```python
from build123d import *

# Parameters (mm, degrees)
SKETCH_13_W         = 280
SKETCH_13_H         = 14.842907488
EXTRUDE_14_DEPTH    = 20
SKETCH_13_W_2       = 18.151554109
SKETCH_13_H_2       = 185
EXTRUDE_14_2_DEPTH  = 20
SKETCH_13_H_3       = 15.157092512
EXTRUDE_14_3_DEPTH  = 20
SKETCH_13_W_3       = 16.848445891
EXTRUDE_14_4_DEPTH  = 20
SKETCH_29_W         = 18.151554109
SKETCH_29_H         = 14.842907488
SKETCH_29_W_2       = 16.848445891
SKETCH_29_H_2       = 15.157092512
EXTRUDE_15_DEPTH    = 400
EXTRUDE_START       = -16.848446
SKETCH_33_W         = 13.5
SKETCH_33_H         = 185
EXTRUDE_16_DEPTH    = 16.848446
EXTRUDE_START_2     = -18.151554
SKETCH_32_W         = 13.5
SKETCH_32_H         = 185
EXTRUDE_17_DEPTH    = 18.151554
EXTRUDE_START_3     = -14.842907
SKETCH_31_W         = 280
SKETCH_31_H         = 13.5
EXTRUDE_18_DEPTH    = 14.842907
SKETCH_30_W         = 280
SKETCH_30_H         = 13.5
EXTRUDE_19_DEPTH    = 15.15709
SKETCH_34_R         = 7
CUT_EXTRUDE_1_DEPTH = 20


with BuildPart() as part:
    # Sketch 13 → Extrude 14 (new body)
    with BuildSketch(Plane.XY):
        with Locations((158.151554109, 207.578546256)):
            Rectangle(SKETCH_13_W, SKETCH_13_H)
    extrude(amount=EXTRUDE_14_DEPTH)



with BuildPart() as body_2:
    # Sketch 13 → Extrude 14 2 (new body)
    with BuildSketch(Plane.XY):
        with Locations((9.075777055, 107.657092512)):
            Rectangle(SKETCH_13_W_2, SKETCH_13_H_2)
    extrude(amount=EXTRUDE_14_2_DEPTH)


with BuildPart() as body_3:
    # Sketch 13 → Extrude 14 3 (new body)
    with BuildSketch(Plane.XY):
        with Locations((158.151554109, 7.578546256)):
            Rectangle(SKETCH_13_W, SKETCH_13_H_3)
    extrude(amount=EXTRUDE_14_3_DEPTH)


with BuildPart() as body_4:
    # Sketch 13 → Extrude 14 4 (new body)
    with BuildSketch(Plane.XY):
        with Locations((306.575777055, 107.657092512)):
            Rectangle(SKETCH_13_W_3, SKETCH_13_H_2)
    extrude(amount=EXTRUDE_14_4_DEPTH)


with BuildPart() as part_1:
    add(part.part)

    add(body_2.part)  # Extrude 15 merges body 2

    add(body_3.part)  # Extrude 15 merges body 3

    add(body_4.part)  # Extrude 15 merges body 4
    # Sketch 29 → Extrude 15 (add)
    with BuildSketch(Plane.XY):
        with Locations((9.075777055, 207.578546256)):
            Rectangle(SKETCH_29_W, SKETCH_29_H)
        with Locations((306.575777055, 207.578546256)):
            Rectangle(SKETCH_29_W_2, SKETCH_29_H)
        with Locations((9.075777055, 7.578546256)):
            Rectangle(SKETCH_29_W, SKETCH_29_H_2)
        with Locations((306.575777055, 7.578546256)):
            Rectangle(SKETCH_29_W_2, SKETCH_29_H_2)
    extrude(amount=EXTRUDE_15_DEPTH)

    # Sketch 33 → Extrude 16 (add)
    with BuildSketch(Plane(origin=(315, 0, 0), x_dir=(0, 0, -1), z_dir=(1, 0, 0)).offset(EXTRUDE_START)):
        with Locations((-323.114974864, 107.657092512)):
            Rectangle(SKETCH_33_W, SKETCH_33_H)
    extrude(amount=EXTRUDE_16_DEPTH)

    # Sketch 32 → Extrude 17 (add)
    with BuildSketch(Plane.ZY.offset(EXTRUDE_START_2)):
        with Locations((323.114974864, 107.657092512)):
            Rectangle(SKETCH_32_W, SKETCH_32_H)
    extrude(amount=EXTRUDE_17_DEPTH)

    # Sketch 31 → Extrude 18 (add)
    with BuildSketch(Plane(origin=(0, 215, 0), x_dir=(1, 0, 0), z_dir=(0, 1, 0)).offset(EXTRUDE_START_3)):
        with Locations((158.151554109, -345.610164736)):
            Rectangle(SKETCH_31_W, SKETCH_31_H)
    extrude(amount=EXTRUDE_18_DEPTH)

    # Sketch 30 → Extrude 19 (add)
    with BuildSketch(Plane.XZ):
        with Locations((158.151554109, 345.610164736)):
            Rectangle(SKETCH_30_W, SKETCH_30_H)
    extrude(amount=-EXTRUDE_19_DEPTH)

    # Sketch 34 → Cut-Extrude 1 (cut)
    with BuildSketch(Plane(origin=(0, 0, 0), x_dir=(-1, 0, 0), z_dir=(0, 0, -1))):
        with Locations((-279.91, 207.578546256)):
            Circle(SKETCH_34_R)
        with Locations((-279.91, 7.566753944)):
            Circle(SKETCH_34_R)
        with Locations((-28.27, 207.578546256)):
            Circle(SKETCH_34_R)
        with Locations((-28.27, 7.566753944)):
            Circle(SKETCH_34_R)
    extrude(amount=-CUT_EXTRUDE_1_DEPTH, mode=Mode.SUBTRACT)


solid = part_1.part
```
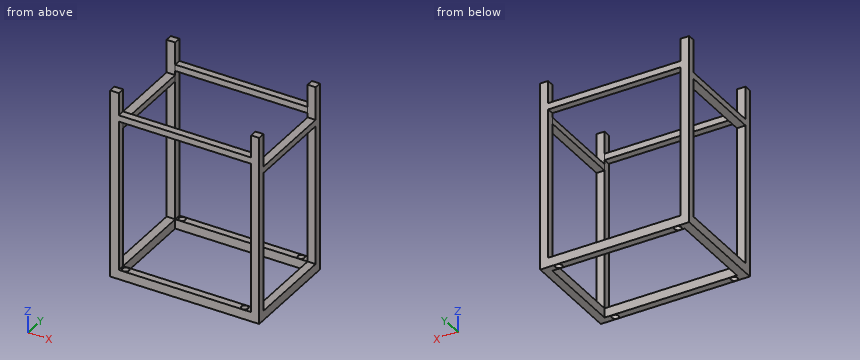
Source: CAD feature listing. Evaluate the final solid. Frame: model axes, mm. Round coordinates to 2 decimals unless told otherwise and drop trailing zeros. Loops run counter-clockwise (first coordinate to the right, second up) from the corner with the lowest first, then second, coordinate; pieces in that order, holes last. Notation, with made-up numbers: M 36.5,3 L 77.5,3 A20 cw 77.5,27 Z; hole C 26.5,-15.5 d3. An arc over 180 degrees is marked long. Use a Markdown table: item, result. Add a question column.
1. Cut plane A-A, the plane x = 28.27. Output: boundary loops of the cut face in (y, z), and give its area (3 significant figures).
2. Cut plane C-C, the plane y = 97.5. Output: boundary loops of the cut face in (x, z), and give its area (3 significant figures).
3. Ray query, line 1 along Y through (x, z) = (28.27, 6.5); line 2 along Y through (x, z) = (284.5, 352); line 3 along Z through (x, y) = (191.5, 14.5). Return the intervals inside material, ascending. Write a range as [from, to].
4. Cut plane B-B, the plane z = 245. Output: boundary loops of the cut face in (x, y).
5. Contact query for flat-ended pins moving along their axis: pin 1 (12 mm diameter, centred on x = 136, y = 6.5, fed in from +Z); pin 2 (5 mm diameter, centred on x = 309.5, y = 110.5, fed in from +Z) (3 decimals). Output: stop coordinate, or through.
Solution:
| question | item | result |
|---|---|---|
| 1 | outline | M 0,0 L 0.57,0 L 0.57,20 L 0,20 Z; M 0,338.86 L 15.16,338.86 L 15.16,352.36 L 0,352.36 Z; M 14.57,0 L 15.16,0 L 15.16,20 L 14.57,20 Z; M 200.16,0 L 200.58,0 L 200.58,20 L 200.16,20 Z; M 200.16,338.86 L 215,338.86 L 215,352.36 L 200.16,352.36 Z; M 214.58,0 L 215,0 L 215,20 L 214.58,20 Z |
| 1 | area | 445 mm2 |
| 2 | outline | M 0,0 L 18.15,0 L 18.15,20 L 0,20 Z; M 0,316.36 L 18.15,316.36 L 18.15,329.86 L 0,329.86 Z; M 298.15,0 L 315,0 L 315,20 L 298.15,20 Z; M 298.15,316.36 L 315,316.36 L 315,329.86 L 298.15,329.86 Z |
| 2 | area | 1,170 mm2 |
| 3 | line 1 | y = [0, 0.57], [14.57, 15.16], [200.16, 200.58], [214.58, 215] |
| 3 | line 2 | y = [0, 15.16], [200.16, 215] |
| 3 | line 3 | z = [0, 20], [338.86, 352.36] |
| 4 | outline | M 0,0 L 18.15,0 L 18.15,15.16 L 0,15.16 Z; M 0,200.16 L 18.15,200.16 L 18.15,215 L 0,215 Z; M 298.15,0 L 315,0 L 315,15.16 L 298.15,15.16 Z; M 298.15,200.16 L 315,200.16 L 315,215 L 298.15,215 Z |
| 5 | pin 1 | stops at z = 352.36 |
| 5 | pin 2 | stops at z = 329.865 |
